Autodesk Inventor part; units mm, degrees
ref_plane "YZ Plane" through (0, 0, 0) normal (1, 0, 0) x (0, 1, 0)
ref_plane "XZ Plane" through (0, 0, 0) normal (0, 1, 0) x (-1, 0, 0)
ref_plane "XY Plane" through (0, 0, 0) normal (0, 0, 1) x (1, 0, 0)
sketch "Esquisse1" plane through (0, 0, 0) normal (0, 1, 0) x (-1, 0, 0)
  line L0 (0, 0) -> (150, 0)
  line L1 (150, 0) -> (150, -150)
  line L2 (150, -150) -> (0, -150)
  line L3 (0, -150) -> (0, 0)
  dimension "d0" = 150
  dimension "d1" = 150
extrude "Extrusion1" add sketch "Esquisse1" along normal blind 3
sketch "Esquisse2" plane through (0, 0, 0) normal (1, 0, 0) x (0, 0, -1)
  line L0 (0, 0) -> (35, 0)
  line L1 (35, 0) -> (35, -9)
  line L2 (0, -9) -> (0, 0)
  line L3 (22.4477, -3.1) -> (12.5523, -3.1)
  arc A0 (25.2, -9) -> (22.4477, -3.1) centre (17.5, -9) ccw
  arc A1 (12.5523, -3.1) -> (9.8, -9) centre (17.5, -9) ccw
  line L4 (25.2, -9) -> (35, -9)
  line L5 (9.8, -9) -> (0, -9)
  point P0 (17.4477, 0)
  point P1 (7.5523, 0)
  point P2 (5.9342, -9)
  point P3 (22.4477, 0)
  point P4 (12.5523, 0)
  dimension "d4" = 35
  dimension "d5" = 9
extrude "Extrusion2" add sketch "Esquisse2" against normal blind 18.6
ref_plane "Plan de construction1" through (-150, 3, -4.9) normal (0, 0, 1) x (1, 0, 0)
ref_plane "Plan de construction2" through (0, -9, -30.1) normal (0, 0, -1) x (-1, 0, 0)
ref_plane "Plan de construction3" through (-4.5, 3, 0) normal (1, 0, 0) x (0, 0, -1)
ref_plane "Plan de construction4" through (-14.1, 3, 0) normal (1, 0, 0) x (0, 0, -1)
hole "Perçage1" at (-14.1, -9, -30.1) direction (0, 1, 0) diameter 6.3 depth 8.1
hole "Perçage2" at (-4.5, -9, -30.1) direction (0, 1, 0) diameter 6.3 depth 8.1
hole "Perçage3" at (-4.5, -9, -4.9) direction (0, 1, 0) diameter 6.3 depth 8.1
hole "Perçage4" at (-14.1, -9, -4.9) direction (0, 1, 0) diameter 6.3 depth 8.1
pattern_linear "Réseau rectangulaire1" count 2 spacing 115 along (0, 0, -1) count 2 spacing 131.4 along (-1, 0, 0) of "Extrusion2", "Perçage2", "Perçage1", "Perçage3", "Perçage4"
sketch "Esquisse5" plane through (0, 0, 0) normal (0, -1, 0) x (1, 0, 0)
  line L0 (-18.6, -5) -> (-38.6, -5)
  line L1 (-38.6, -5) -> (-38.6, -30)
  line L2 (-38.6, -30) -> (-18.6, -30)
  line L3 (-18.6, -30) -> (-18.6, -5)
  circle A0 centre (-23.1, -9.5) radius 2.3
  circle A1 centre (-23.1, -25.5) radius 2.3
  point P0 (0, 0)
  dimension "d61" = 20
  dimension "d62" = 25
  dimension "d63" = 4.6
  dimension "d64" = 4.6
extrude "Extrusion4" add sketch "Esquisse5" along normal blind 5.7
pattern_linear "Réseau rectangulaire2" count 2 spacing 115 along (0, 0, -1) of "Extrusion4"
ref_plane "Plan de construction5" through (-75, 3, 0) normal (1, 0, 0) x (0, 0, -1)
mirror "Mise en miroir1" about plane through (-75, 3, 0) normal (1, 0, 0) of "Extrusion4", "Réseau rectangulaire2"
ref_plane "Plan de construction6" through (-131.4, 0, -9.5) normal (0, 0, 1) x (1, 0, 0)
properties part number "plateauV2102"
The model under review builds one solid part; all positions refer to its coordinate system, in mm. A direction names the side the tool comes from. Round coordinates to 2 decimals unless told otherwise and drop trailing zeros. Loops run counter-clockwise (first coordinate to the right, second up) from the corner with the lowest first, then second, coordinate; pieces in that order, holes last. Notation, with made-up numbers: (-16.5, 79.25) - (31.5, 79.25) arc R30 ccw to (31.5, 102.25) - close; hole circle Ø7 at (25, 71). An arc over 180 degrees is marked (long way). Use CSV: the item, a comma, the result in double quotes.
(1) Clearance check with flat-ended pins moving along their axes: P1, Ø4.5, axis at y = -2.5, z = -136, coming from the +X side; P2, Ø7.5, axis at x = -23.1, z = -25.5, coming from the -Y side; P3, Ø1.5, axis at x = -46, z = -26.5, coming from the -Y side; P4, Ø3, axis at x = -26, y = -4, coming from the -Z side. State where each tip first meets the part, or that it passes through.
Working result:
P1,"stops at x = 0"
P2,"stops at y = -5.7"
P3,"stops at y = 0"
P4,"stops at z = -145"
(2) Take a section at A-A, the plane x = -126.9. Give the boundary of the cut face in (y, z).
Working result:
outline,"(-5.7, -145) - (0, -145) - (0, -150) - (3, -150) - (3, 0) - (0, 0) - (0, -5) - (-5.7, -5) - (-5.7, -7.2) - (0, -7.2) - (0, -11.8) - (-5.7, -11.8) - (-5.7, -23.2) - (0, -23.2) - (0, -27.8) - (-5.7, -27.8) - (-5.7, -30) - (0, -30) - (0, -120) - (-5.7, -120) - (-5.7, -122.2) - (0, -122.2) - (0, -126.8) - (-5.7, -126.8) - (-5.7, -138.2) - (0, -138.2) - (0, -142.8) - (-5.7, -142.8) - close"
(3) Take a section at C-C, the plane x = -45. Give the boundary of the cut face in (y, z), plus the area to 3 significant figures.
Working result:
outline,"(0, -150) - (3, -150) - (3, 0) - (0, 0) - close"
area,"450 mm^2"
(4) Take a section at B-B, the plane z = -53. Give the boundary of the cut face in (x, y), plus the area to 3 significant figures.
Working result:
outline,"(-150, 0) - (0, 0) - (0, 3) - (-150, 3) - close"
area,"450 mm^2"
(5) For line 1 (X direction, y = -5.75, z = -119.9); line 2 (Z direction, x = -145.5, y = -3); line 3 (X direction, y = -6, z = -119), list the stretches that pass through material, from the lowest coordinate up.
Working result:
line 1,"x = -150 to -148.65, -142.35 to -139.05, -132.75 to -131.4, -18.6 to -17.25, -10.95 to -7.65, -1.35 to 0"
line 2,"z = -150 to -148.25, -141.95 to -123.05, -116.75 to -115, -35 to -33.25, -26.95 to -8.05, -1.75 to 0"
line 3,"x = -150 to -148.52, -142.48 to -138.92, -132.88 to -131.4, -18.6 to -17.12, -11.08 to -7.52, -1.48 to 0"
(6) The part is to be moulded in two halves that separate along X. For faces 5 (the flat face through (0, 1, -74)), 6 (the flat face through (-141, -9, -120)), 7 (the flat face through (-14, -0.9, -5)), say which applies: pulls with the +X half, pulls with the -X half, needs draft (parallel to the pull), parting line crosses it, or undercut.
Working result:
face 5,"pulls with the +X half"
face 6,"needs draft"
face 7,"undercut"
(7) Machinability: for faces 1 (the cylindrical face through (-9.17, -5.702, -125.542)), 2 (the flat face through (-18.6, -5, -4)), 3 (the flat face through (-38.6, -3, -17)), 4 (the cylindrical face through (-11.025, -4.893, -29.417)), which of the approach directions +Z, -Z, +X, -X, +Y, -Y give a long, thin tool a straight path to every point of the face, cutting with its end or side? Answer none if there is none.
Working result:
face 1,"+X, -Y"
face 2,"+Z, -Y"
face 3,"+Z, -Z, -Y"
face 4,"-Y"
